Work out the finished part from the listing and answer in its coordinate system (mm). Round coordinates to 2 decimals unless told otherwise and drop trailing zeros. Order: outer loops, then holes, each group sorted by start corner. A loop starts at its lowest first (then second) coordinate and runs counter-clockwise, first axis right, second up. Notation, with made-up numbers: (58.25, -20.5) - (117.25, -20.5) arc R18 ccw to (117.25, 5.5) - close; hole circle Ø2 at (79.25, -23.5). An arc over 180 degrees is marked (long way). Use CSV: the item, a comma, the result in double quotes.
from build123d import *

# Parameters (mm, degrees)
F1_DEPTH = 28.5
F2_D     = 2.6
F4_D     = 4.4


with BuildPart() as f1:
    # F0 (on Front) → F1 (new body)
    with BuildSketch(Plane.XZ):
        with BuildLine():
            ThreePointArc((1.3, 2.1354156504), (2.1794494718, 1.2247448714), (2.5, 0))
            Line((2.5, 0), (2.5, 45))
            Line((2.5, 45), (1.3, 45))
            Line((1.3, 45), (1.3, 2.1354156504))
        make_face()
        with BuildLine():
            ThreePointArc((1.3, 2.1354156504), (-2.1794494718, -1.2247448714), (2.5, 0))
            ThreePointArc((2.5, 0), (2.1794494718, 1.2247448714), (1.3, 2.1354156504))
        make_face()
    extrude(amount=-F1_DEPTH)

    # F2 (through all)
    with Locations(Plane.XZ):
        with Locations((0, 0)):
            Hole(F2_D / 2)

    # F4 (through all)
    with Locations(Plane.YZ.offset(2.5)):
        with Locations((14.25, 39.8), (22.25, 30.4), (6.25, 30.4), (14.25, 17)):
            Hole(F4_D / 2)


solid = f1.part
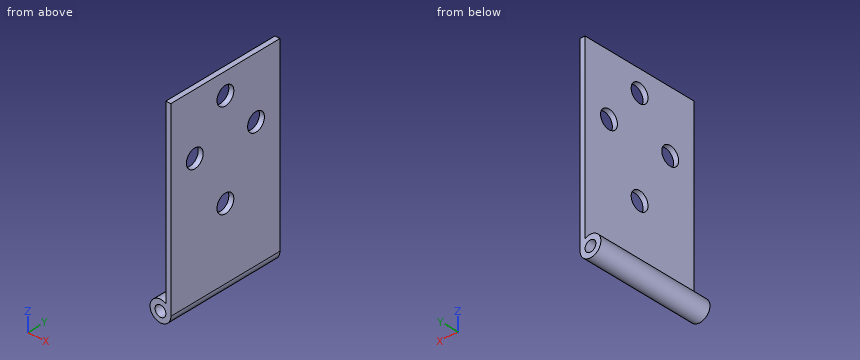
(1) Each of these flat-tipped pins is pushed along its axis until it touches: pin 1 (6 mm diameter, centred on y = 4, z = 17.5, fed in from -X); pin 2 (2 mm diameter, centred on x = -1, y = 23.5, fed in from -Z); pin 3 (1.5 mm diameter, centred on x = -1.5, y = 25, fed in from +Z). Where does it stop, or does it pass through?
Findings below:
pin 1,"stops at x = 1.3"
pin 2,"stops at z = -2.5"
pin 3,"stops at z = 2.38"
(2) Find section A-A (y = 14.25). Determine the outline of the cut face in (x, z), and give its area (3 significant figures).
Findings below:
outline,"(1.3, 2.14) arc R2.5 ccw (long way) to (2.5, 0) - (2.5, 14.8) - (1.3, 14.8) - close; (1.3, 19.2) - (2.5, 19.2) - (2.5, 37.6) - (1.3, 37.6) - close; (1.3, 42) - (2.5, 42) - (2.5, 45) - (1.3, 45) - close; hole circle Ø2.6 at (0, 0)"
area,"56.0 mm²"
(3) Find section C-C (y = 22.25). Determine the outline of the cut face in (x, z), and give its area (3 significant figures).
Findings below:
outline,"(1.3, 2.14) arc R2.5 ccw (long way) to (2.5, 0) - (2.5, 28.2) - (1.3, 28.2) - close; (1.3, 32.6) - (2.5, 32.6) - (2.5, 45) - (1.3, 45) - close; hole circle Ø2.6 at (0, 0)"
area,"61.2 mm²"
(4) Find section D-D (z = 30.4). Determine the outline of the cut face in (x, y), and give its area (3 significant figures).
Findings below:
outline,"(1.3, 0) - (2.5, 0) - (2.5, 4.05) - (1.3, 4.05) - close; (1.3, 8.45) - (2.5, 8.45) - (2.5, 20.05) - (1.3, 20.05) - close; (1.3, 24.45) - (2.5, 24.45) - (2.5, 28.5) - (1.3, 28.5) - close"
area,"23.6 mm²"
(5) Find the intervals of material crossed by L1, parallel to Z at x = 2, y = 14.25; L2, parallel to Z at x = 0, y = 6.75; L3, parallel to Z at x = 1.6, y = 14.25, in increasing order. Write a range as from..to.
Findings below:
L1,"z = -1.5..14.8, 19.2..37.6, 42..45"
L2,"z = -2.5..-1.3, 1.3..2.5"
L3,"z = -1.92..14.8, 19.2..37.6, 42..45"
(6) Find section B-B (x = 0). Determine the outline of the cut face in (y, z), and give its area (3 significant figures).
Findings below:
outline,"(0, -2.5) - (28.5, -2.5) - (28.5, -1.3) - (0, -1.3) - close; (0, 1.3) - (28.5, 1.3) - (28.5, 2.5) - (0, 2.5) - close"
area,"68.4 mm²"
